```python
from build123d import *

# Parameters (mm, degrees)
SKETCH1_R           = 1.5
SKETCH1_R_2         = 1.4
BOSS_EXTRUDE1_DEPTH = 2.3
BOSS_EXTRUDE2_START = -1.3
SKETCH1_4_R         = 1.9
SKETCH1_4_R_2       = 1.5
SKETCH1_4_R_3       = 1.4
BOSS_EXTRUDE2_DEPTH = 1.3
SKETCH1_5_R         = 1.4
BOSS_EXTRUDE3_DEPTH = 19
CHAMFER1_SIZE       = 0.5


with BuildPart() as part:
    # Sketch1 → Boss-Extrude1 (new body)
    # profile 1 of 2: a face of its own
    with BuildSketch(Plane(origin=(0, 0, 0), x_dir=(1, 0, 0), z_dir=(0, 1, 0))):
        with Locations(Location((0, 0, 0), (0, 0, 270))):
            Circle(SKETCH1_R)
        Circle(SKETCH1_R_2, mode=Mode.SUBTRACT)
    # profile 2 of 2: a face of its own
    with BuildSketch(Plane(origin=(0, 0, 0), x_dir=(1, 0, 0), z_dir=(0, 1, 0))):
        Circle(SKETCH1_R_2)
    extrude(amount=BOSS_EXTRUDE1_DEPTH)

    # Sketch1<4> → Boss-Extrude2 (add)
    # profile 1 of 3: a face of its own
    with BuildSketch(Plane(origin=(0, 0, 0), x_dir=(1, 0, 0), z_dir=(0, 1, 0)).offset(BOSS_EXTRUDE2_START)):
        with Locations(Location((0, 0, 0), (0, 0, 270))):
            Circle(SKETCH1_4_R)
        with Locations(Location((0, 0, 0), (0, 0, 270))):
            Circle(SKETCH1_4_R_2, mode=Mode.SUBTRACT)
    # profile 2 of 3: a face of its own
    with BuildSketch(Plane(origin=(0, 0, 0), x_dir=(1, 0, 0), z_dir=(0, 1, 0)).offset(BOSS_EXTRUDE2_START)):
        with Locations(Location((0, 0, 0), (0, 0, 270))):
            Circle(SKETCH1_4_R_2)
        Circle(SKETCH1_4_R_3, mode=Mode.SUBTRACT)
    # profile 3 of 3: a face of its own
    with BuildSketch(Plane(origin=(0, 0, 0), x_dir=(1, 0, 0), z_dir=(0, 1, 0)).offset(BOSS_EXTRUDE2_START)):
        Circle(SKETCH1_4_R_3)
    extrude(amount=BOSS_EXTRUDE2_DEPTH)

    # Sketch1<5> → Boss-Extrude3 (add)
    with BuildSketch(Plane(origin=(0, 0, 0), x_dir=(1, 0, 0), z_dir=(0, 1, 0))):
        with Locations(Location((0, 0, 0), (0, 0, 270))):
            Circle(SKETCH1_5_R)
    extrude(amount=-BOSS_EXTRUDE3_DEPTH)

    # Chamfer1
    chamfer1_edges = [part.edges().sort_by_distance(p)[0] for p in [
        (0, -1.3, -1.4),
    ]]
    chamfer(chamfer1_edges, length=CHAMFER1_SIZE - 0.0001)  # a hair under: the kernel refuses the full size


solid = part.part
```
Build history of the part. All positions in model axes, mm. A direction names the side the tool comes from. Coordinates: 2 decimals unless noted, no trailing zeros. Write each loop counter-clockwise with the first axis right and the second up, starting at its lowest first coordinate (ties: lowest second). Pieces come first, ordered by that corner, then holes.
1. Band-saw the part on C-C, the plane y = -16.5. Give the cut face in (x, z).
Answer block:
outline: circle Ø2.8 at (0, 0)
2. 3-axis set-ups, long thin cutter, end or side, ignore diameter. For faces 1 (the cylindrical face through (0.45, 1.13, 1.43)), 2 (the cylindrical face through (0.06, -10.28, -1.4)), 3 (the flat face through (0, 2.3, 0)): which of +Z, -Z, +X, -X, +Y, -Y reach the whole face in a straight line?
Answer block:
face 1: +Y
face 2: -Y
face 3: +Z, -Z, +X, -X, +Y
3. Drill centre lines: probe 1 along X at (y, z) = (-7, 0.05); probe 2 along X at (y, z) = (-8.25, 0.9). Where is each one in solid material? Low to high.
Answer block:
probe 1: x = -1.4 to 1.4
probe 2: x = -1.07 to 1.07
4. Drop flat-ended pins along their axis: pin 1 (1 mm diameter, centred on y = -15.5, z = -1, fed in from -X); pin 2 (1.5 mm diameter, centred on x = 1, y = -14.5, fed in from -Z). Give the stop position or say it passes through.
Answer block:
pin 1: stops at x = -1.31
pin 2: stops at z = -1.38
